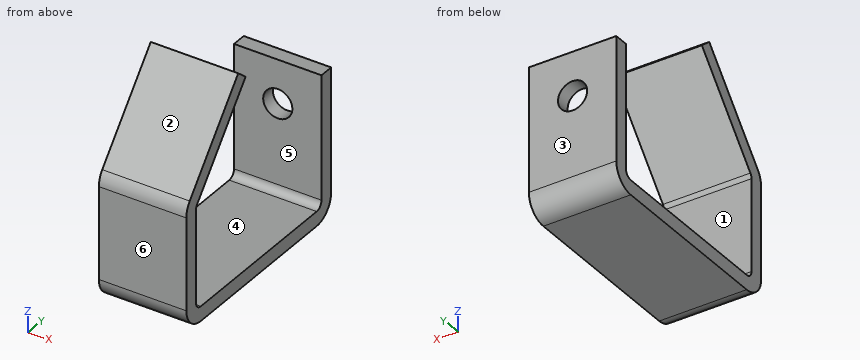
from build123d import *

# Parameters (mm, degrees)
BASE_EXTRUDE_THIN_DEPTH = 19.05
CUT_EXTRUDE1_REACH      = 132.7
SKETCH2_R               = 6.35


with BuildPart() as part:
    # Sketch1 → Base-Extrude-Thin (new, symmetric)
    with BuildSketch(Plane(origin=(0, 0, 0), x_dir=(0, 0, -1), z_dir=(1, 0, 0))):
        with BuildLine():
            Line((-83.36505771, 32.653610572), (-45.335245167, 0.742808893))
            ThreePointArc((-45.335245167, 0.742808893), (-44.380308461, 0.191475929), (-43.294394506, 0))
            Line((-43.294394506, 0), (-3.175, 0))
            ThreePointArc((-3.175, 0), (-0.92993597, 0.92993597), (0, 3.175))
            Line((0, 3.175), (0, 79.375))
            ThreePointArc((0, 79.375), (-0.92993597, 81.62006403), (-3.175, 82.55))
            Line((-3.175, 82.55), (-57.15, 82.55))
            Line((-57.15, 82.55), (-57.15, 88.9))
            Line((-57.15, 88.9), (-3.175, 88.9))
            ThreePointArc((-3.175, 88.9), (3.560192091, 86.110192091), (6.35, 79.375))
            Line((6.35, 79.375), (6.35, 3.175))
            ThreePointArc((6.35, 3.175), (3.560192091, -3.560192091), (-3.175, -6.35))
            Line((-3.175, -6.35), (-43.294394506, -6.35))
            ThreePointArc((-43.294394506, -6.35), (-46.552136371, -5.775572213), (-49.416946488, -4.121573321))
            Line((-49.416946488, -4.121573321), (-87.446759032, 27.789228358))
            Line((-87.446759032, 27.789228358), (-83.36505771, 32.653610572))
        make_face()
    extrude(amount=BASE_EXTRUDE_THIN_DEPTH, both=True)

    # Sketch2 → Cut-Extrude1 (cut, up to next)
    with BuildSketch(Plane(origin=(0, 88.9, 0), x_dir=(-1, 0, 0), z_dir=(0, 1, 0)), mode=Mode.PRIVATE) as cut_extrude1_sk1:
        with Locations(Location((0, 38.1, 0), (0, 0, 90))):
            Circle(SKETCH2_R)
    cut_extrude1_tool1 = extrude(cut_extrude1_sk1.sketch, amount=-CUT_EXTRUDE1_REACH, mode=Mode.PRIVATE) & part.part
    add(cut_extrude1_tool1.solids().sort_by_distance((0, 88.9, 38.1))[0], mode=Mode.SUBTRACT)


solid = part.part
Could you check a few things on this model? Use its own coordinates, in mm. Face numbers are marked on the shaded views. A direction names the side the tool comes from. Give positions to 0.01 mm unless a question says otherwise; leave off trailing zeros. Order: outer loops, then holes, each group sorted by start corner. A loop starts at its lowest first (then second) coordinate and runs counter-clockwise, first axis right, second up. Notation, with made-up numbers: (3.5, 76) - (27.5, 76) arc R17 cw to (27.5, 104) - close; hole circle Ø7 at (62.25, 24.5). An arc over 180 degrees is marked (long way). Return JSON: item names as keys, results as strings. Group by question number.
Q1. Suppose I cut it at B-B, the plane z = 12.5. Please give me the cut outline in (x, y), and give its area (3 significant figures).
Q2. Please list where these lines run through material, in increasing order: line 1 along X through (y, z) = (86.25, 38.1); line 2 along Y through (x, z) = (-4, 26); line 3 along Z through (x, y) = (-14, 10.5). Write a range as [from, to].
Q3. Thinking about a two-plate mould opening in Y: for the marked faces 1, 2 and 3, which applies, pulls with the +Y half, pulls with the -Y half, needs draft (parallel to the pull), parting line crosses it, or undercut?
Q4. Suppose I cut it at D-D, the plane x = -13. Please give me the cut outline in (y, z) (3 decimals), and give its area (3 significant figures).
Q5. Suppose I cut it at C-C, the plane z = 38.1. Please give me the cut outline in (x, y).
Q6. Suppose I cut it at A-A, the plane x = 0. Please give me the cut outline in (y, z) (3 decimals).
Q7. Which directions (+Z, -Z, +X, -X, +Y, -Y) give clear straight access to the entire face, cutting with the end or side of a thin tool? Please do the marked faces 4, 5 and 6.
Q8. Will these pins go through, and if not, where does the flat tip stop? pin 1 Ø1.9 at (x, y) = (0, 86.5) entering from +Z; pin 2 Ø19 at (x, y) = (-5.5, 60) entering from +Z; pin 3 Ø8 at (x, z) = (-8.5, 74) entering from -Y; pin 4 Ø4 at (x, z) = (-5, 59) entering from +Y.
Resolved:
{
 "1": {"outline": "(-19.05, -6.35) - (19.05, -6.35) - (19.05, 0) - (-19.05, 0) - close; (-19.05, 82.55) - (19.05, 82.55) - (19.05, 88.9) - (-19.05, 88.9) - close", "area": "484 mm2"},
 "2": {"line 1": "x = [-19.05, -6.35], [6.35, 19.05]", "line 2": "y = [-6.35, 0], [82.55, 88.9]", "line 3": "z = [-6.35, 0], [56.96, 66.84]"},
 "3": {"face 1": "undercut", "face 2": "pulls with the -Y half", "face 3": "pulls with the +Y half"},
 "4": {"outline": "(-6.35, 3.175) arc R9.525 ccw to (3.175, -6.35) - (79.375, -6.35) arc R9.525 ccw to (88.9, 3.175) - (88.9, 57.15) - (82.55, 57.15) - (82.55, 3.175) arc R3.175 cw to (79.375, 0) - (3.175, 0) arc R3.175 cw to (0, 3.175) - (0, 43.294) arc R3.175 cw to (0.743, 45.335) - (32.654, 83.365) - (27.789, 87.447) - (-4.122, 49.417) arc R9.525 ccw to (-6.35, 43.294) - close", "area": "1,550 mm2"},
 "5": {"outline": "(-19.05, -6.35) - (19.05, -6.35) - (19.05, 0) - (-19.05, 0) - close; (-19.05, 82.55) - (-6.35, 82.55) - (-6.35, 88.9) - (-19.05, 88.9) - close; (6.35, 82.55) - (19.05, 82.55) - (19.05, 88.9) - (6.35, 88.9) - close"},
 "6": {"outline": "(-6.35, 3.175) arc R9.525 ccw to (3.175, -6.35) - (79.375, -6.35) arc R9.525 ccw to (88.9, 3.175) - (88.9, 31.75) - (82.55, 31.75) - (82.55, 3.175) arc R3.175 cw to (79.375, 0) - (3.175, 0) arc R3.175 cw to (0, 3.175) - (0, 43.294) arc R3.175 cw to (0.743, 45.335) - (32.654, 83.365) - (27.789, 87.447) - (-4.122, 49.417) arc R9.525 ccw to (-6.35, 43.294) - close; (82.55, 44.45) - (88.9, 44.45) - (88.9, 57.15) - (82.55, 57.15) - close"},
 "7": {"face 4": "+X, -X", "face 5": "+Z, +X, -X", "face 6": "+Z, -Z, +X, -X, -Y"},
 "8": {"pin 1": "stops at z = 57.15", "pin 2": "stops at z = 0", "pin 3": "stops at y = 13.15", "pin 4": "stops at y = 88.9"}
}
